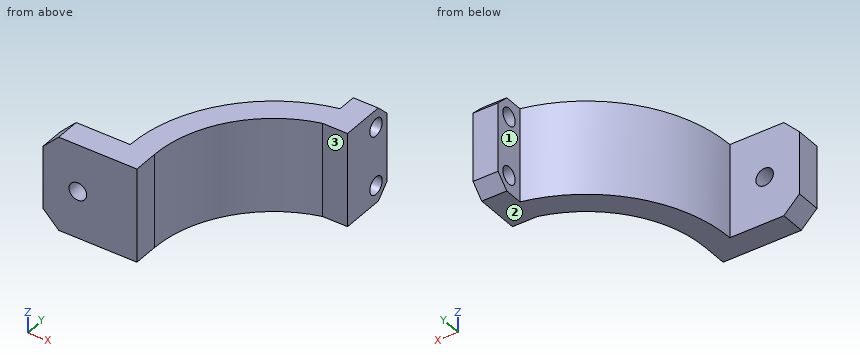
```python
from build123d import *

# Parameters (mm, degrees)
BOSS_EXTRUDE1_DEPTH = 15
CHAMFER1_SIZE       = 2.5
SKETCH2_R           = 1.4
CUT_EXTRUDE1_DEPTH  = 15
CHAMFER2_SIZE       = 2
SKETCH3_R           = 1.4
CUT_EXTRUDE2_DEPTH  = 47.129659115


with BuildPart() as part:
    # Sketch1 → Boss-Extrude1 (new body)
    with BuildSketch(Plane.XY):
        with BuildLine():
            Line((-19, 0), (-19, -4))
            Line((-19, -4), (-34, -4))
            Line((-34, -4), (-34, 0))
            Line((-34, 0), (-22.883234523, 0))
            ThreePointArc((-22.883234523, 0), (-17.861391251, 14.304304416), (-5, 22.33030278))
            Line((-5, 22.33030278), (-5, 27.33030278))
            Line((-5, 27.33030278), (-1, 27.33030278))
            Line((-1, 27.33030278), (-1, 18.33030278))
            Line((-1, 18.33030278), (-5, 18.33030278))
            ThreePointArc((-5, 18.33030278), (-15.099668871, 11.532562595), (-19, 0))
        make_face()
    extrude(amount=BOSS_EXTRUDE1_DEPTH)

    # Chamfer1
    chamfer1_edges = [part.edges().sort_by_distance(p)[0] for p in [
        (-34, -2, 0),
        (-34, -2, 15),
    ]]
    chamfer(chamfer1_edges, length=CHAMFER1_SIZE)

    # Sketch2 → Cut-Extrude1 (cut)
    with BuildSketch(Plane.ZY.offset(5)):
        with Locations(Location((2.8, 24.83030278, 0), (0, 0, 270))):
            Circle(SKETCH2_R)
        with Locations(Location((12.2, 24.83030278, 0), (0, 0, 270))):
            Circle(SKETCH2_R)
    extrude(amount=-CUT_EXTRUDE1_DEPTH, mode=Mode.SUBTRACT)

    # Chamfer2
    chamfer2_edges = [part.edges().sort_by_distance(p)[0] for p in [
        (-3, 27.33030278, 0),
        (-3, 27.33030278, 15),
    ]]
    chamfer(chamfer2_edges, length=CHAMFER2_SIZE)

    # Sketch3 → Cut-Extrude2 (cut, through all)
    with BuildSketch(Plane(origin=(0, 0, 0), x_dir=(1, 0, 0), z_dir=(0, 1, 0))):
        with Locations(Location((-28.441617262, -7.5, 0), (0, 0, 270))):
            Circle(SKETCH3_R)
    extrude(amount=-CUT_EXTRUDE2_DEPTH, mode=Mode.SUBTRACT)


solid = part.part
```
Check sheet for the modelled part. Datum: model origin and axes. Units: mm. Face numbers are marked on the shaded views. A direction names the side the tool comes from. Coordinates: 2 decimals unless noted, no trailing zeros. Order: outer loops, then holes, each group sorted by start corner. A loop starts at its lowest first (then second) coordinate and runs counter-clockwise, first axis right, second up. Notation, with made-up numbers: (-0.5, 49.25) -> (19.5, 49.25) arc R17 cw to (19.5, 75.25) -> close; hole circle Ø1 at (42.5, -6.5). An arc over 180 degrees is marked (long way). Write item = value, one per line. Start each with the question number.
1) Material ranges on L1, parallel to X at y = -1.25, z = 7.5; L2, parallel to Y at x = -26, z = 6.25; L3, parallel to X at y = 0.5, z = 4.25, recorded low to high.
2) Cross-section at B-B (z = 5.25). Enter the section's corners in (x, y).
3) Go/stop test with flat-tipped pins: P1, Ø4.5, axis at x = -2.5, z = 4.5, coming from the -Y side; P2, Ø2, axis at x = -19.5, z = 2, coming from the +Y side; P3, Ø2, axis at y = 24.83, z = 12.2, coming from the +X side; P4, Ø6, axis at y = 19.5, z = 2, coming from the -X side. Record where each tip stops, or that it passes through.
4) Access from +Z, -Z, +X, -X, +Y, -Y to the whole of each face (thin tool, end or side, straight path). Record for the marked faces 1, 2 and 3.
5) Cross-section at C-C (y = 23). Enter the section's corners in (x, z), then the cut area to 3 significant figures.
6) Cross-section at A-A (z = 7.5). Enter the section's corners in (x, y), then the cut area to 3 significant figures.
7) Cross-section at D-D (x = -14). Enter the section's corners in (y, z), then the cut area to 3 significant figures.
Ans:
q1.L1 = -34 to -29.84, -27.04 to -19
q1.L2 = -4 to 0
q1.L3 = -22.88 to -18.99
q2.outline = (-34, -4) -> (-19, -4) -> (-19, 0) arc R19 cw to (-5, 18.33) -> (-1, 18.33) -> (-1, 27.33) -> (-5, 27.33) -> (-5, 22.33) arc R22.88 ccw to (-22.88, 0) -> (-34, 0) -> close
q3.P1 = 18.33
q3.P2 = 13.47
q3.P3 = through
q3.P4 = -15.86
q4.face_1 = +Z, -Z, -X, +Y
q4.face_2 = -Z, +X, -X, +Y, -Y
q4.face_3 = +Z, -Z, +X, -Y
q5.outline = (-5, 0) -> (-1, 0) -> (-1, 15) -> (-5, 15) -> close
q5.area = 60.0 mm²
q6.outline = (-34, -4) -> (-29.84, -4) -> (-29.84, 0) -> (-34, 0) -> close; (-27.04, -4) -> (-19, -4) -> (-19, 0) arc R19 cw to (-5, 18.33) -> (-1, 18.33) -> (-1, 27.33) -> (-5, 27.33) -> (-5, 22.33) arc R22.88 ccw to (-22.88, 0) -> (-27.04, 0) -> close
q6.area = 193 mm²
q7.outline = (12.85, 0) -> (18.1, 0) -> (18.1, 15) -> (12.85, 15) -> close
q7.area = 78.8 mm²
